Here's how the part is built. I have some questions about the finished solid (model axes, mm). Face numbers are marked on the shaded views. Coordinates: 2 decimals unless noted, no trailing zeros. Order: outer loops, then holes, each group sorted by start corner. A loop starts at its lowest first (then second) coordinate and runs counter-clockwise, first axis right, second up. Notation, with made-up numbers: (-21.5, 76.5) - (17.5, 76.5) arc R5 cw to (17.5, 83.5) - close; hole circle Ø2 at (51, -30). An arc over 180 degrees is marked (long way). Answer as CSV lines item,"result". Start each with the question number.
Item 1: Imagine slicing it at B-B on y = 4. List the corners of the cut face in (x, z) for me.
Item 2: Imagine slicing it at C-C on x = 5.3. List the corners of the cut face in (y, z) for me, and give its area (3 significant figures).
Item 3: I'm going to push flat-ended pins straight in: pin 1 (6 mm diameter, centred on x = 1, z = 7, fed in from +Y); pin 2 (1.5 mm diameter, centred on x = -5, y = 14.5, fed in from +Z). Where does each tip first touch, or does it pass through?
Item 4: Imagine slicing it at A-A on z = 5. List the corners of the cut face in (x, y) for me, and give its area (3 significant figures).
Item 5: We'd pull the mould along Z, two halves only. Please class the marked faces 1, 2 and 3: pulls with the +Z half, pulls with the -Z half, needs draft (parallel to the pull), parting line crosses it, or undercut.
Item 6: I need wall thicknesses on line 1 (X direction, y = 1, z = 0); line 2 (Z direction, x = -0.25, y = 5.75); line 3 (Z direction, x = 1, y = 4.75). Which ranges of each line are inside material? Lowest first, please.
Item 7: Imagine slicing it at D-D on y = 15.75. List the corners of the cut face in (x, z) for me, and give its area (3 significant figures).
from build123d import *

# Parameters (mm, degrees)
SCHIZZO2_W                   = 12.5
SCHIZZO2_H                   = 12.5
SCHIZZO2_R                   = 0.15
ESTRUSIONE_ESTRUSIONE1_DEPTH = 8
SCHIZZO3_R                   = 3
TAGLIO_ESTRUSIONE1_DEPTH     = 18.102631376
SCHIZZO4_R                   = 0.75
TAGLIO_ESTRUSIONE2_DEPTH     = 3.5
SCHIZZO5_R                   = 4
ESTRUSIONE_ESTRUSIONE2_DEPTH = 10
SMUSSO1_SIZE                 = 1
FORO_3_8_3_8_1_D             = 3.8
FORO_3_8_3_8_1_DEPTH         = 15
FORO_3_8_3_8_1_TIP           = 1.141635176


with BuildPart() as part:
    # Schizzo1 → Rivoluzione1 (revolve)
    with BuildSketch(Plane.XY, mode=Mode.PRIVATE) as rivoluzione1_sk:
        Polygon((-0.15, 0), (-0.15, -3), (-0.5, -3), (-4, -1), (-4, 0), align=None)
    revolve(rivoluzione1_sk.sketch.rotate(Axis((0, -26.528171736, 0), (0, 1, 0)), 270), axis=Axis((0, -26.528171736, 0), (0, 1, 0)))

    # Schizzo2 → Estrusione-Estrusione1 (add)
    with BuildSketch(Plane(origin=(0, 0, 0), x_dir=(1, 0, 0), z_dir=(0, 1, 0))):
        with Locations((0, -2.25)):
            Rectangle(SCHIZZO2_W, SCHIZZO2_H)
        with Locations(Location((0, 0, 0), (0, 0, 90))):
            Circle(SCHIZZO2_R, mode=Mode.SUBTRACT)
    extrude(amount=ESTRUSIONE_ESTRUSIONE1_DEPTH)

    # Schizzo3 → Taglio-Estrusione1 (cut, through all)
    with BuildSketch(Plane(origin=(6.25, 0, 0), x_dir=(0, 0, -1), z_dir=(1, 0, 0))):
        with Locations((-5, 4)):
            Circle(SCHIZZO3_R)
    extrude(amount=-TAGLIO_ESTRUSIONE1_DEPTH, mode=Mode.SUBTRACT)

    # Schizzo4 → Taglio-Estrusione2 (cut)
    with BuildSketch(Plane(origin=(0, 0, -4), x_dir=(-1, 0, 0), z_dir=(0, 0, -1))):
        with Locations((-5.3, 4)):
            Circle(SCHIZZO4_R)
    extrude(amount=-TAGLIO_ESTRUSIONE2_DEPTH, mode=Mode.SUBTRACT)

    # Schizzo5 → Estrusione-Estrusione2 (add)
    with BuildSketch(Plane(origin=(0, 8, 0), x_dir=(1, 0, 0), z_dir=(0, 1, 0))):
        with Locations(Location((0, 0, 0), (0, 0, 90))):
            Circle(SCHIZZO5_R)
    extrude(amount=ESTRUSIONE_ESTRUSIONE2_DEPTH)

    # Smusso1
    smusso1_edges = [part.edges().sort_by_distance(p)[0] for p in [
        (0, 18, 4),
    ]]
    chamfer(smusso1_edges, length=SMUSSO1_SIZE)

    # Foro Ø3.8 (3.8)-1
    with Locations(Plane(origin=(0, 18, 0), x_dir=(1, 0, 0), z_dir=(0, 1, 0))):
        with Locations((0, 0)):
            Hole(FORO_3_8_3_8_1_D / 2, depth=FORO_3_8_3_8_1_DEPTH)
            with Locations((0, 0, -(FORO_3_8_3_8_1_DEPTH + FORO_3_8_3_8_1_TIP / 2))):  # 118° drill point
                Cone(0, FORO_3_8_3_8_1_D / 2, FORO_3_8_3_8_1_TIP, mode=Mode.SUBTRACT)


solid = part.part
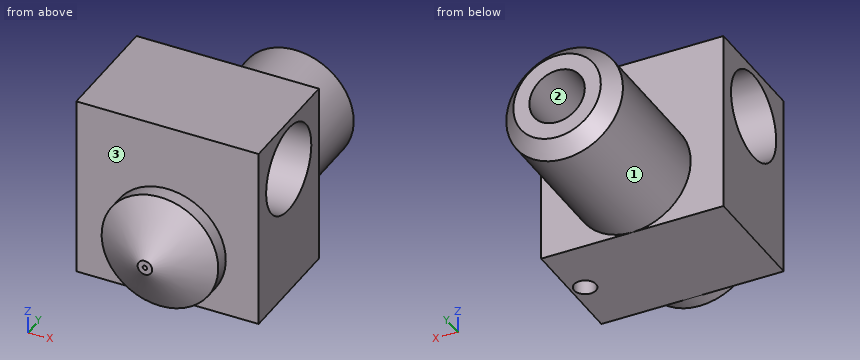
Responses:
1,outline,"(-6.25, -4) - (4.55, -4) - (4.55, -0.5) - (6.05, -0.5) - (6.05, -4) - (6.25, -4) - (6.25, 2) - (-6.25, 2) - close; (-6.25, 8) - (6.25, 8) - (6.25, 8.5) - (-6.25, 8.5) - close; hole circle Ø3.8 at (0, 0)"
2,outline,"(0, -4) - (3.25, -4) - (3.25, -0.5) - (4.75, -0.5) - (4.75, -4) - (8, -4) - (8, 8.5) - (0, 8.5) - close; hole circle Ø6 at (4, 5)"
2,area,"66.5 mm^2"
3,pin 1,"stops at y = 8"
3,pin 2,"passes through"
4,outline,"(-6.25, 0) - (6.25, 0) - (6.25, 1) - (-6.25, 1) - close; (-6.25, 7) - (6.25, 7) - (6.25, 8) - (-6.25, 8) - close"
4,area,"25.0 mm^2"
5,face 1,"parting line crosses it"
5,face 2,"undercut"
5,face 3,"needs draft"
6,line 1,"x = -6.25 to -0.15, 0.15 to 6.25"
6,line 2,"z = -4 to -1.88, 1.88 to 2.56, 7.44 to 8.5"
6,line 3,"z = -4 to -1.62, 1.62 to 2.1, 7.9 to 8.5"
7,outline,"circle Ø8 at (0, 0); hole circle Ø3.8 at (0, 0)"
7,area,"38.9 mm^2"
